Here's how the part is built. I have some questions about the finished solid (model axes, mm). A direction names the side the tool comes from. Give positions to 0.01 mm unless a question says otherwise; leave off trailing zeros. Write each loop counter-clockwise with the first axis right and the second up, starting at its lowest first coordinate (ties: lowest second). Pieces come first, ordered by that corner, then holes. Notation, with made-up numbers: (5, 20.5) - (22, 20.5) arc R25 ccw to (22, 33.5) - close; hole circle Ø5 at (31, 59.25). An arc over 180 degrees is marked (long way). One line per item, written item: value. Start each with the question number.
1) Please list where these lines run through material, in increasing order: L1, parallel to X at y = 6, z = 6.75; L2, parallel to Y at x = -23, z = 0; L3, parallel to Z at x = -25.5, y = -5. Write a range as [from, to].
2) Imagine slicing it at A-A on y = 9.5. Write out the boundary of the cut face in (x, z).
3) On a 3-axis mill with a long thin cutter (end or side, diameter ignored), from which of +Z, -Z, +X, -X, +Y, -Y can I reach the whole of each face in a straight line? I mean faces 1 (the cylindrical face through (-22.434, 7.597, -0.026)), 2 (the cylindrical face through (-22.43, -2.82, -3.36)), 3 (the cylindrical face through (-22.455, -0.136, -0.26)). Say none if no direction works.
4) We'd pull the mould along X, two halves only. Please class faces 4 (the cylindrical face through (-16.624, 7.324, -7.142)), 5 (the flat face through (-15.864, 4, 2)), 6 (the cylindrical face through (-22.434, 3.599, -5.477)): +X half, -X half, draft (parallel to the pull), parting line (faces both ways), or undercut.
5) Imagine slicing it at D-D on y = 6.5. Write out the boundary of the cut face in (x, z), plus the area to 3 significant figures.
6) Imagine slicing it at B-B on z = -0.5. Write out the boundary of the cut face in (x, y).
7) I'm going to push flat-ended pins straight in: P1, Ø4, axis at x = -26.5, y = -2, coming from the -Z side (3 decimals); P2, Ø1.5, axis at x = -18.5, y = 5, coming from the +Z side; P3, Ø1, axis at x = -18, z = -0.5, coming from the -Y side; P4, Ø2.5, axis at y = 1.85, z = 0, coming from the -X side. Where does each tip first touch, or does it pass through?
from build123d import *

# Parameters (mm, degrees)
SKETCH_3_R               = 2
CUT_EXTRUDE_2_DEPTH      = 17
SKETCH_4_W               = 2.5
SKETCH_4_H               = 2.683329606
CUT_EXTRUDE_3_DEPTH      = 17
PATTERN_CIRCULAR_1_COUNT = 15
EXTRUDE_START            = 1.5
SKETCH_5_R               = 9
SKETCH_5_R_2             = 2
EXTRUDE_1_DEPTH          = 1.5
SKETCH_6_R               = 9
SKETCH_6_R_2             = 2
EXTRUDE_2_DEPTH          = 1.5


with BuildPart() as part:
    # 草图1 → 旋转2 (revolve)
    with BuildSketch(Plane.XY, mode=Mode.PRIVATE) as revolve_2_sk:
        Polygon((-27.363734917, 8.847191366), (-27.363734917, 3.847191366), (-28.613734917, 3.847191366), (-28.613734917, 1.847191366), (-16.113734917, 1.847191366), (-16.113734917, 3.847191366), (-17.363734917, 3.847191366), (-17.363734917, 8.847191366), align=None)
    revolve(revolve_2_sk.sketch.rotate(Axis((-48.964491856, 1.847191366, 0), (1, 0, 0)), 90), axis=Axis((-48.964491856, 1.847191366, 0), (1, 0, 0)))

    # 草图3 → 切除-拉伸2 (cut)
    with BuildSketch(Plane.ZY.offset(28.613734917)):
        with Locations((0, 1.847191366)):
            Circle(SKETCH_3_R)
    extrude(amount=-CUT_EXTRUDE_2_DEPTH, mode=Mode.SUBTRACT)

    # 草图4 → 切除-拉伸3 (cut)
    with BuildSketch(Plane.ZY.offset(27.363734917)):
        with Locations((0, 10.188856169)):
            Rectangle(SKETCH_4_W, SKETCH_4_H)
        with BuildLine():
            Line((1.25, 8.847191366), (-1.25, 8.847191366))
            ThreePointArc((-1.25, 8.847191366), (0, 7.597191366), (1.25, 8.847191366))
        make_face()
    cut_extrude_3 = extrude(amount=-CUT_EXTRUDE_3_DEPTH, mode=Mode.SUBTRACT)

    # 阵列(圆周)1: 切除-拉伸3 ×15 about axis
    pattern_circular_1_axis = Axis((0, 1.847191366, 0), (1, 0, 0))
    for i in range(1, PATTERN_CIRCULAR_1_COUNT):
        add(cut_extrude_3.rotate(pattern_circular_1_axis, i * 360 / PATTERN_CIRCULAR_1_COUNT), mode=Mode.SUBTRACT)

    # 草图5 → 凸台-拉伸1 (add)
    with BuildSketch(Plane.ZY.offset(27.363734917).offset(EXTRUDE_START)):
        with Locations((0, 1.847191366)):
            Circle(SKETCH_5_R)
        with Locations((0, 1.847191366)):
            Circle(SKETCH_5_R_2, mode=Mode.SUBTRACT)
    extrude(amount=-EXTRUDE_1_DEPTH)

    # 草图6 → 凸台-拉伸2 (add)
    with BuildSketch(Plane(origin=(-17.363734917, 0, 0), x_dir=(0, 0, -1), z_dir=(1, 0, 0))):
        with Locations(Location((0, 1.847191366, 0), (0, 0, 180))):
            Circle(SKETCH_6_R)
        with Locations(Location((0, 1.847191366, 0), (0, 0, 180))):
            Circle(SKETCH_6_R_2, mode=Mode.SUBTRACT)
    extrude(amount=EXTRUDE_2_DEPTH)


solid = part.part
Numbers:
1. L1: [-28.86, -27.36], [-17.36, -15.86]
1. L2: [-5.15, -0.15], [3.85, 7.6]
1. L3: [-0.21, 0.21]
2. outline: (-28.86, -4.74) - (-27.36, -4.74) - (-27.36, 4.74) - (-28.86, 4.74) - close; (-17.36, -4.74) - (-15.86, -4.74) - (-15.86, 4.74) - (-17.36, 4.74) - close
3. face 1: +Y
3. face 2: none
3. face 3: +X, -X
4. face 4: draft
4. face 5: +X half
4. face 6: undercut
5. outline: (-28.86, -7.7) - (-27.36, -7.7) - (-27.36, -3.95) - (-17.36, -3.95) - (-17.36, -7.7) - (-15.86, -7.7) - (-15.86, 7.7) - (-17.36, 7.7) - (-17.36, 3.95) - (-27.36, 3.95) - (-27.36, 7.7) - (-28.86, 7.7) - close
5. area: 125 mm^2
6. outline: (-28.86, -7.14) - (-27.36, -7.14) - (-27.36, -4.19) - (-17.36, -4.19) - (-17.36, -7.14) - (-15.86, -7.14) - (-15.86, -0.09) - (-28.86, -0.09) - close; (-28.86, 3.78) - (-15.86, 3.78) - (-15.86, 10.83) - (-17.36, 10.83) - (-17.36, 7.7) - (-27.36, 7.7) - (-27.36, 10.83) - (-28.86, 10.83) - close
7. P1: z = -8.765
7. P2: z = 6.17
7. P3: y = -5.15
7. P4: through
